Could you check a few things on this model? Use its own coordinates, in mm. Face numbers are marked on the shaded views. A direction names the side the tool comes from. Give positions to 0.01 mm unless a question says otherwise; leave off trailing zeros. Loops run counter-clockwise (first coordinate to the right, second up) from the corner with the lowest first, then second, coordinate; pieces in that order, holes last. Notation, with made-up numbers: (-35.5, 82.25) - (17.5, 82.25) arc R29 cw to (17.5, 104.25) - close; hole circle Ø3 at (-3, 52). An arc over 180 degrees is marked (long way). Write each question's results on one line, items separated by ' | '. Start each with the question number.
```python
from build123d import *

# Parameters (mm, degrees)
F0_R      = 38.195919
F1_DEPTH  = 350
F2_R      = 25.71702
F3_DEPTH  = 45
F4_R      = 15.726109
F5_DEPTH  = 200
F6_R      = 2
F7_R      = 7.719414
F8_DEPTH  = 25
F9_R      = 21.707928
F10_DEPTH = 80
F11_R     = 14.568553
F12_DEPTH = 75
F13_R     = 9.827947
F14_DEPTH = 25


with BuildPart() as f1:
    # F0 (on Front) → F1 (new body)
    with BuildSketch(Plane.XZ):
        Circle(F0_R)
    extrude(amount=F1_DEPTH)

    # F2 (on face) → F3 (join)
    with BuildSketch(Plane(origin=(0, 0, 0), x_dir=(-1, 0, 0), z_dir=(0, 1, 0))):
        Circle(F2_R)
    extrude(amount=F3_DEPTH)

    # F4 (on face) → F5 (join)
    with BuildSketch(Plane(origin=(0, 45, 0), x_dir=(-1, 0, 0), z_dir=(0, 1, 0))):
        Circle(F4_R)
    extrude(amount=F5_DEPTH)

    # F6
    f6_edges = [f1.edges().sort_by_distance(p)[0] for p in [
        (15.726109, 245, 0),
        (25.71702, 45, 0),
        (-38.195919, 0, 0),
    ]]
    fillet(f6_edges, radius=F6_R)

    # F7 (on face) → F8 (join)
    with BuildSketch(Plane(origin=(0, 245, 0), x_dir=(-1, 0, 0), z_dir=(0, 1, 0))):
        Circle(F7_R)
    extrude(amount=F8_DEPTH)

    # F9 (on face) → F10 (join)
    with BuildSketch(Plane.XZ.offset(350)):
        Circle(F9_R)
    extrude(amount=F10_DEPTH)

    # F11 (on face) → F12 (join)
    with BuildSketch(Plane.XZ.offset(430)):
        Circle(F11_R)
    extrude(amount=F12_DEPTH)

    # F13 (on face) → F14 (join)
    with BuildSketch(Plane.XZ.offset(505)):
        Circle(F13_R)
    extrude(amount=F14_DEPTH)


solid = f1.part
```
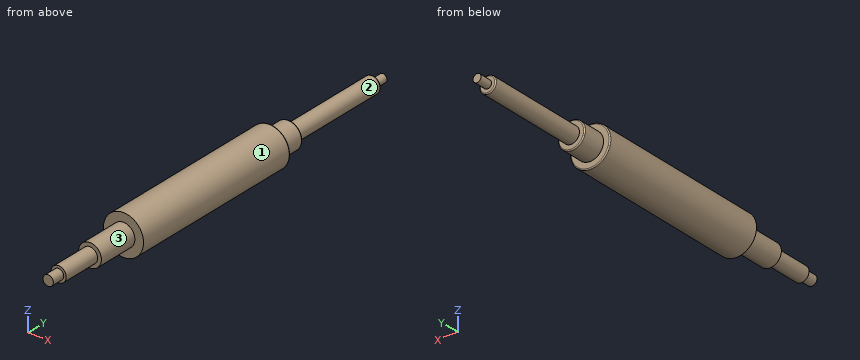
Q1. I want a section at C-C, the plane y = -467.5. List the corners of the cut face in (x, z) for me, then the cut area to 3 significant figures.
Q2. I want a section at D-D, the plane y = -207. List the corners of the cut face in (x, z) for me.
Q3. I need wall thicknesses on L1, parallel to Y at x = 27.5, z = 0; L2, parallel to Y at x = 9.5, z = -8.5; L3, parallel to Z at x = 1.5, y = -380. Which ranges of each line are inside material? Lowest first, please. Write a range as from..to.
Q4. Which directions (+Z, -Z, +X, -X, +Y, -Y) give clear straight access to the entire face, cutting with the end or side of a thin tool? Please do the marked faces 1, 2 and 3.
Q5. I'm going to push flat-ended pins straight in: pin 1 Ø4 at (x, y) = (29, -104.5) entering from -Z; pin 2 Ø1.5 at (x, z) = (-14.5, -2.5) entering from +Y; pin 3 Ø6 at (y, z) = (-104, -15) entering from +X. Where does each tip first touch, or does it pass through?
Conclusion:
1) outline: circle Ø29.14 at (0, 0) | area: 667 mm^2
2) outline: circle Ø76.39 at (0, 0)
3) L1: -350..0 | L2: -505..245 | L3: -21.66..21.66
4) face 1: +Y, -Y | face 2: +Y | face 3: -Y
5) pin 1: z = -27.02 | pin 2: y = 244.99 | pin 3: x = 36.26
